Autodesk Inventor part; units mm, degrees
ref_plane "YZ Plane" through (0, 0, 0) normal (1, 0, 0) x (0, 1, 0)
ref_plane "XZ Plane" through (0, 0, 0) normal (0, 1, 0) x (-1, 0, 0)
ref_plane "XY Plane" through (0, 0, 0) normal (0, 0, 1) x (1, 0, 0)
sketch "Sketch2" plane through (0, 0, 0) normal (1, 0, 0) x (0, 1, 0)
  line L0 (55, 30) -> (58, 30)
  line L1 (58, 30) -> (58, 20)
  line L2 (58, 20) -> (55, 20)
  line L3 (15, 55) -> (15, 58)
  line L4 (15, 58) -> (5, 58)
  line L5 (5, 58) -> (5, 55)
  line L6 (55, 30) -> (55, 55)
  line L7 (15, 55) -> (55, 55)
  line L8 (55, 20) -> (55, 8)
  line L9 (55, 8) -> (58, 8)
  arc A0 (54.5719, 1.4376) -> (56.0607, -1.0607) centre (55, 0) ccw
  line L10 (57, -5) -> (51.9134, -5)
  line L11 (56.5709, 2.033) -> (54.5719, 1.4376)
  line L12 (56.2929, -0.8284) -> (56.0607, -1.0607)
  line L13 (58, 8) -> (58, 3.9497)
  line L14 (58, -1.5355) -> (58, -4)
  arc A1 (56.5709, 2.033) -> (58, 3.9497) centre (56, 3.9497) ccw
  arc A2 (58, -1.5355) -> (56.2929, -0.8284) centre (57, -1.5355) ccw
  arc A3 (57, -5) -> (58, -4) centre (57, -4) ccw
  line L15 (-25, 54) -> (-25, 46.6369)
  arc A4 (-20.9, 53.2) -> (-18.701, 52.75) centre (-20, 52) ccw
  line L16 (-20.9, 53.2) -> (-20.9, 53.2)
  line L17 (-19.134, 53.5) -> (-18.701, 52.75)
  line L18 (5, 55) -> (-18.2679, 55)
  line L19 (-21.5, 55) -> (-24, 55)
  arc A5 (-18.2679, 55) -> (-19.134, 53.5) centre (-18.2679, 54) ccw
  arc A6 (-25, 46.6369) -> (-22.1154, 44.8432) centre (-23, 46.6369) ccw
  arc A7 (-24, 55) -> (-25, 54) centre (-24, 54) ccw
  arc A8 (-20.9, 53.2) -> (-21.5, 55) centre (-21.5, 54) ccw
  arc A9 (49.9167, -2.8846) -> (47.1154, 16.7374) centre (0, 0) ccw
  arc A10 (16.7374, 47.1154) -> (-22.1154, 44.8432) centre (0, 0) ccw
  line L20 (47, 17.4069) -> (47, 37)
  line L21 (17.4069, 47) -> (37, 47)
  arc A11 (47, 37) -> (37, 47) centre (37, 37) ccw
  arc A12 (49.9167, -2.8846) -> (51.9134, -5) centre (51.9134, -3) ccw
  arc A13 (16.7374, 47.1154) -> (17.4069, 47) centre (17.4069, 49) ccw
  arc A14 (47, 17.4069) -> (47.1154, 16.7374) centre (49, 17.4069) ccw
  point P0 (-25, 43.3013)
  point P1 (58, -5)
  point P2 (-25, 55)
  point P3 (49.7494, -5)
  point P4 (49.7494, -5)
  point P5 (17.0587, 47)
  point P6 (47, 17.0587)
  dimension "d5" = 10
  dimension "d6" = 10
  dimension "d13" = 40
  dimension "d14" = 25
  dimension "d15" = 3
  dimension "d16" = 3
  dimension "d22" = 55
  dimension "d23" = 55
  dimension "d43" = 12
  dimension "d44" = 3
  dimension "d46" = 3
  dimension "d48" = 3
  dimension "d53" = 2
  dimension "d54" = 1
  dimension "d57" = 80
  dimension "d58" = 3
  dimension "d59" = 5
  dimension "d61" = 3
  dimension "d64" = 1
  dimension "d65" = 2
  dimension "d66" = 1
  dimension "d67" = 3
  dimension "d75" = 4.0503
  dimension "d76" = 60
  dimension "d78" = 5
  dimension "d79" = 3
  dimension "d87" = 60
  dimension "d92" = 8
  dimension "d93" = 50
  dimension "d94" = 50
  dimension "d95" = 8
  dimension "d96" = 10
  dimension "d97" = 2
  dimension "d98" = 2
extrude "Extrusion3" add sketch "Sketch2" along normal blind 3
properties part number "OpenROV 2_3 Dev Tube Brace"
CAD build for the part. Positions are in the model's coordinates, mm. A direction names the side the tool comes from. Give positions to 0.01 mm unless a question says otherwise; leave off trailing zeros. Write each loop counter-clockwise with the first axis right and the second up, starting at its lowest first coordinate (ties: lowest second). Pieces come first, ordered by that corner, then holes. Notation, with made-up numbers: M -16.75,52.5 L 10.25,52.5 A34 cw 10.25,89.5 Z; hole C 21,-12 d3. An arc over 180 degrees is marked long. Put each result on its own line as item: value. Start each with the question number.
(1) Band-saw the part on A-A, the plane z = 18.5. Write the cut outline in (x, y).
(2) Flat gauge pins, fed straight in: pin 1 Ø0.9 at (x, z) = (1, 56) entering from +Y; pin 2 Ø1.2 at (x, y) = (1.5, -22.5) entering from +Z; pin 3 Ø0.9 at (x, y) = (1.5, 56.5) entering from +Z. Where does each tip first touch, or does it go through?
(3) Which spindle directions (+Z, -Z, +X, -X, +Y, -Y) get a long thin tool onto all of the face, cutting with end or side? Do faces 4 (the face through (1.48, 49.48, 7.2)), 5 (the face through (1, 35, 55)), 6 (the face through (1, 55, 14)), 7 (the face through (1, -6, 55)). Say none if no direction does.
(4) Mould opens along Z. For faces 1 (the face through (1.48, -20.25, 50.52)), 2 (the face through (3, 32, 48)), 3 (the face through (1.479, -3.198, 49.898)) say: +Z half, -Z half, draft (parallel to the pull), parting line (faces both ways), or undercut.
(5) Band-saw the part on B-B, the plane y = -5. Write the cut outline in (x, z), and give its area (3 significant figures).
(6) Probe L1, parallel to Z at x = 2.35, y = 26.5; L2, parallel to Y at x = 1.95, z = 0. List the from-to ranges inside material, lowest first.
Response values:
1. outline: M 0,47 L 3,47 L 3,55 L 0,55 Z
2. pin 1: stops at y = 15
2. pin 2: stops at z = 55
2. pin 3: stops at z = 30
3. face 4: +X, -X, -Y
3. face 5: +Z, +X, -X, +Y
3. face 6: +X, -X, +Y
3. face 7: +Z, +X, -X, -Y
4. face 1: undercut
4. face 2: draft
4. face 3: -Z half
5. outline: M 0,49.75 L 3,49.75 L 3,55 L 0,55 Z
5. area: 15.8 mm2
6. L1: z = 47 to 55
6. L2: y = 50 to 53.5
